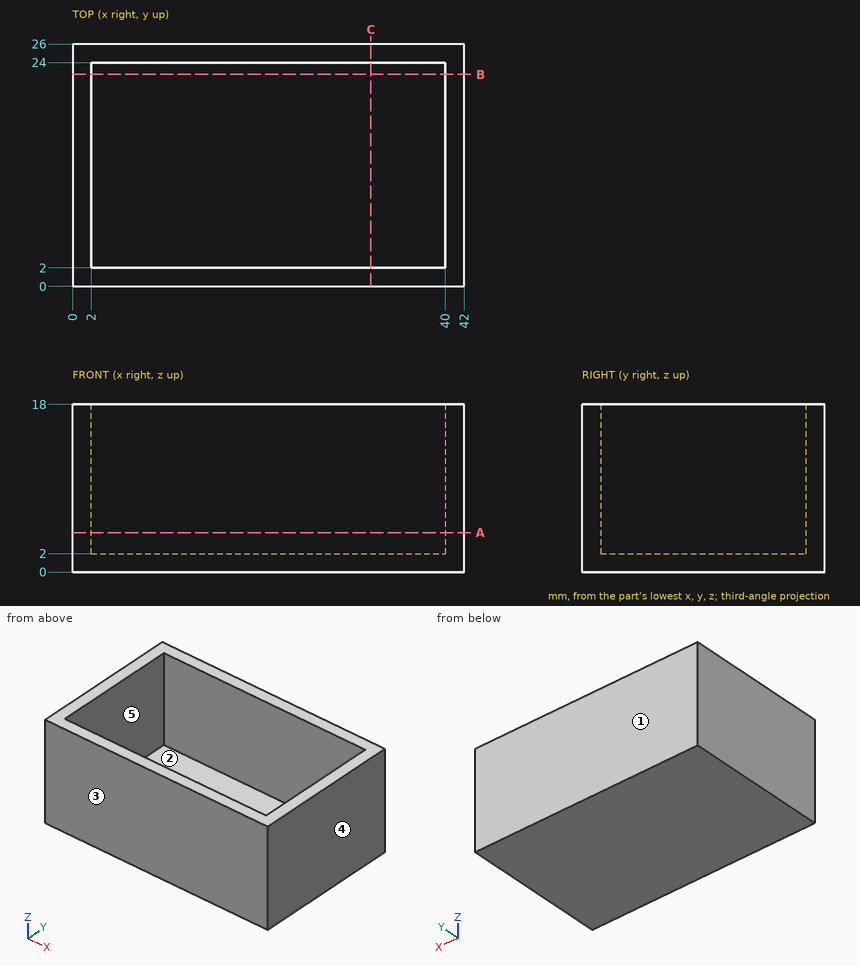
Answer from the drawing. Dimensions are ordinates in mm from the lowest x, y and z of the part. A direction names the side the tool comes from. Give positions to 0.01 mm unless a question says otherwise; leave off trailing zeros. Write each loop counter-clockwise with the first axis right and the second up, starting at its lowest first coordinate (ties: lowest second). Pieces come first, ordered by that corner, then holes. Notation, with made-up numbers: (49.5, 33) -> (63.5, 33) arc R9 ccw to (63.5, 47) -> close; hole circle Ø4 at (-13, 44). An arc over 180 degrees is marked (long way). One line per question, with ' | ' between items. Start each with the question number.
1. Section C-C (x = 32) is taken. Determine the outline of the cut face in (y, z), plus the area to 3 significant figures.
2. Section B-B (y = 22.75) is taken. Determine the outline of the cut face in (x, z).
3. For the marked faces 1 and 2, determine the directions among +Z, -Z, +X, -X, +Y, -Y from which every point of the face is accessible in a straight line to the end or side of a thin tool.
4. For a pull along Y with two mould halves and no side action, classify the marked faces 3, 4 and 5 as pulls with the +Y half, pulls with the -Y half, needs draft (parallel to the pull), parting line crosses it, or undercut.
5. Section A-A (z = 4.25) is taken. Determine the outline of the cut face in (x, y), plus the area to 3 significant figures.
6. Find the intervals of material crossed by probe 1 along X at (y, z) = (7.75, 8.75); probe 2 along Y at (x, z) = (2.5, 7); probe 3 along Z at (x, y) = (9, 2.5), in increasing order.
Response values:
1) outline: (0, 0) -> (26, 0) -> (26, 18) -> (24, 18) -> (24, 2) -> (2, 2) -> (2, 18) -> (0, 18) -> close | area: 116 mm2
2) outline: (0, 0) -> (42, 0) -> (42, 18) -> (40, 18) -> (40, 2) -> (2, 2) -> (2, 18) -> (0, 18) -> close
3) face 1: +Z, -Z, +X, -X, +Y | face 2: +Z
4) face 3: pulls with the -Y half | face 4: needs draft | face 5: undercut
5) outline: (0, 0) -> (42, 0) -> (42, 26) -> (0, 26) -> close; hole (2, 2) -> (40, 2) -> (40, 24) -> (2, 24) -> close | area: 256 mm2
6) probe 1: 0 to 2, 40 to 42 | probe 2: 0 to 2, 24 to 26 | probe 3: 0 to 2
